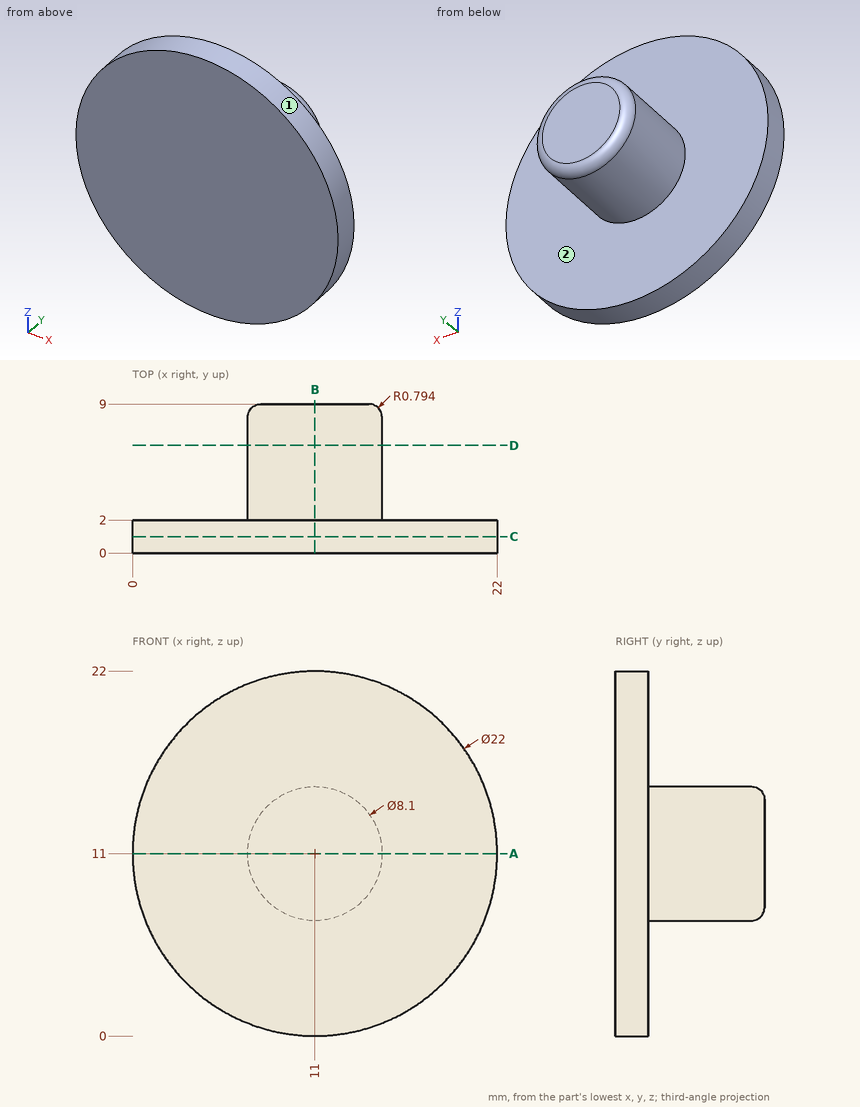
Print and shaded views of the part. All mm, measured from the part's lowest x, y and z. A direction names the side the tool comes from. Coordinates: 2 decimals unless noted, no trailing zeros. Loops run counter-clockwise (first coordinate to the right, second up) from the corner with the lowest first, then second, coordinate; pieces in that order, holes last. Notation, with made-up numbers: (-36, 3) - (-18, 3) arc R21 ccw to (-18, 39) - close; hole circle Ø4 at (-21.5, 39). An arc over 180 degrees is marked (long way). Use one line per item in the form item = value. Start each with the question number.
1) Drill centre lines: L1, parallel to Y at x = 8, z = 14; L2, parallel to X at y = 8.25, z = 7.75 (1 decimal); L3, parallel to Z at x = 13, y = 6.75. Where is each one in solid material? Low to high. Write a range as from..to.
2) Flat gauge pins, fed straight in: pin 1 (4 mm diameter, centred on x = 12.5, y = 8, fed in from -Z); pin 2 (3 mm diameter, centred on y = 6.5, z = 5, fed in from -X); pin 3 (2 mm diameter, centred on x = 6.5, y = 4, fed in from +Z). Where does each tip first touch, or does it go through?
3) Band-saw the part on D-D (y = 6.5). Give the cut face in (x, z).
4) Band-saw the part on B-B (x = 11). Give the cut face in (y, z), and give its area (3 significant figures).
5) Band-saw the part on A-A (z = 11). Give the cut face in (x, y), and give its area (3 significant figures).
6) Band-saw the part on C-C (y = 1). Give the cut face in (x, z).
7) Tool access for the marked faces 1 and 2: list every direction of +Z, -Z, +X, -X, +Y, -Y with a clear straight run to the whole face (end or side of a thin tool).
Check values:
q1.L1 = 0..2
q1.L2 = 8.6..13.4
q1.L3 = 7.48..14.52
q2.pin_1 = 6.95
q2.pin_2 = through
q2.pin_3 = 13.04
q3.outline = circle Ø8.1 at (11, 11)
q4.outline = (0, 0) - (2, 0) - (2, 6.95) - (8.21, 6.95) arc R0.79 ccw to (9, 7.74) - (9, 14.26) arc R0.79 ccw to (8.21, 15.05) - (2, 15.05) - (2, 22) - (0, 22) - close
q4.area = 100 mm2
q5.outline = (0, 0) - (22, 0) - (22, 2) - (15.05, 2) - (15.05, 8.21) arc R0.79 ccw to (14.26, 9) - (7.74, 9) arc R0.79 ccw to (6.95, 8.21) - (6.95, 2) - (0, 2) - close
q5.area = 100 mm2
q6.outline = circle Ø22 at (11, 11)
q7.face_1 = +Y, -Y
q7.face_2 = +Y
